Input: part model. Units: mm. Frame: model coordinates. Face numbers are marked on the shaded views. A direction names the side the tool comes from. Round coordinates to 2 decimals unless told otherwise and drop trailing zeros. Write each loop counter-clockwise with the first axis right and the second up, starting at its lowest first coordinate (ties: lowest second). Pieces come first, ordered by that corner, then holes. Notation, with made-up numbers: (38.25, -3.5) - (77.25, -3.5) arc R15 cw to (77.25, 7.5) - close; hole circle Ø6 at (4.5, 13). An arc over 180 degrees is marked (long way). Use one line per item in the form item = value.
```python
from build123d import *

# Parameters (mm, degrees)
F1_ANGLE    = 50
F2_SIZE     = 1.5
F3_T2_ANGLE = 53.1281028161


# Not quite as in the source:
# - a fillet or chamfer that OpenCascade refuses, or shapes differently, is made with other operations: its cross-section is extruded or revolved along the edge and cut away or added


with BuildPart() as f1:
    # F0 (on Top) → F1 (revolve)
    with BuildSketch(Plane.XY):
        Polygon((-90, -10), (-100, -10), (-100, 10.7), (-95, 10.7), (-97, 11.7), (-105, 11.7), (-105, -13), (-90, -13), align=None)
    revolve(axis=Axis((0, 3.89609579, 0), (0, 1, 0)), revolution_arc=F1_ANGLE)

    # F2
    f2_edges = [f1.edges().sort_by_distance(p)[0] for p in [
        (-81.567701, -10, 38.035644),
    ]]
    chamfer(f2_edges, length=F2_SIZE)

    # F3: chamfer of 1 x 0.5 on 1 edges, made by hand

    # F3_s1 → F3_t2 (revolve, cut)
    with BuildSketch(Plane(origin=(0, 0, 0), x_dir=(0, 1, 0), z_dir=(0.0272944566, 0, -0.9996274369))):
        Polygon((10.7, -95.5), (11.1472135955, -95.894427191), (10.7, -95), align=None)
    revolve(axis=Axis((0, 10.7, 0), (0, 1, 0)), revolution_arc=F3_T2_ANGLE, mode=Mode.SUBTRACT)


solid = f1.part
```
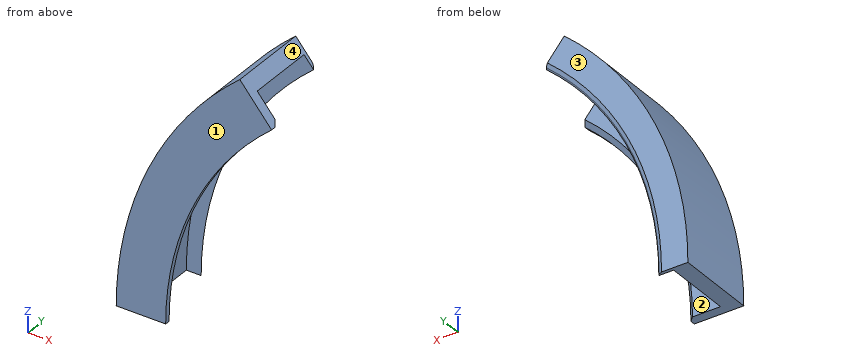
(1) Access query for the marked faces 1 and 2. Directions: +Z, -Z, +X, -X, +Y, -Y. A direction counts if a zero-diameter tool reaches every point of the face in a straight line with its end or side. Return the directions, or none.
Derived:
face_1 = +Z, -Z, +X, -X, -Y
face_2 = -Z, +X
(2) Draft query along Z for the marked faces 3 and 4. Return one class per face: released by +Z, released by -Z, zero draft, split by the parting line, or undercut.
Derived:
face_3 = zero draft
face_4 = released by +Z
(3) Material intervals for L1, parallel to Y at x = -95.5, z = 19; L2, parallel to Y at x = -81, z = 45; L3, parallel to Z at x = -85, y = 9.25, sorted ascending.
Derived:
L1 = -13 to -10, 10.7 to 11.7
L2 = -13 to -10
L3 = 52.68 to 61.64
(4) Cut plane B-B on y = -7. Output: boundary loops of the cut face in (x, z), then the cut area to 3 significant figures.
Derived:
outline = (-105, 0) - (-100, 0) arc R100 cw to (-64.28, 76.6) - (-67.49, 80.43) arc R105 ccw to start
area = 447 mm^2
(5) Cut plane A-A on x = -99. Output: boundary loops of the cut face in (y, z), then the cut area to 3 significant figures.
Derived:
outline = (-13, 0) - (-10, 0) - (-10, 14.11) - (10.7, 14.11) - (10.7, 0) - (11.7, 0) - (11.7, 34.99) - (-13, 34.99) - close
area = 572 mm^2
(6) First-contact query: pin 1 Ø1 at (y, z) = (4, 43.5) entering from -X; pin 2 Ø4 at (y, z) = (2, 38.5) entering from +X; pin 3 Ø12.5 at (x, z) = (-75, 49) entering from +Y. Flat tips, straight axial feed; report the tip coordinate or a pass-through.
Derived:
pin_1 = -95.79
pin_2 = -91.43
pin_3 = 11.08
